For this review, use the dimensioned drawing (mm, ordinates from the lowest corner) and the shaded views. Round coordinates to 2 decimals unless told otherwise and drop trailing zeros. Loops run counter-clockwise (first coordinate to the right, second up) from the corner with the lowest first, then second, coordinate; pieces in that order, holes last. Notation, with made-up numbers: (72, -27.75) -> (112, -27.75) arc R19 ccw to (112, -5.75) -> close; hole circle Ø7 at (37, 70.5). An arc over 180 degrees is marked (long way). Use one line per item in the form item = value. Start each with the question number.
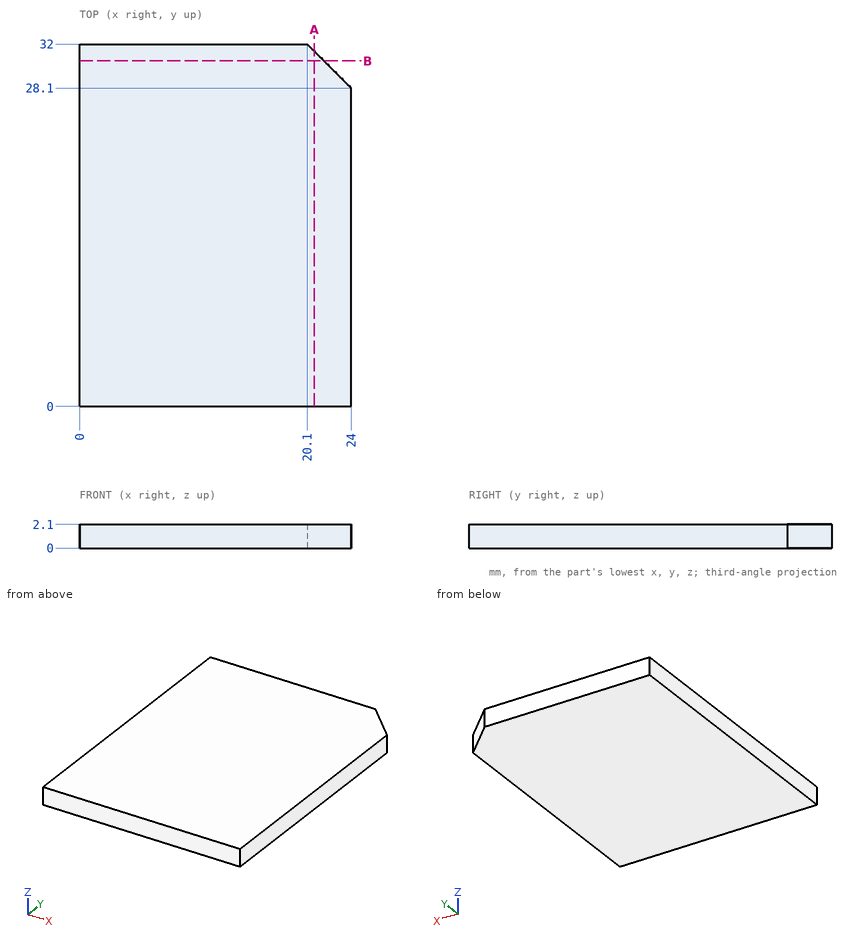
Item 1: Take a section at A-A on x = 20.75. Give the boundary of the cut face in (y, z), plus the area to 3 significant figures.
Item 2: Take a section at B-B on y = 30.5. Give the boundary of the cut face in (x, z).
Item 3: Wall thickness on line 1 (Y direction, x = 22.75, z = 2.05); line 2 (Y direction, x = 22.5, z = 0.3); line 3 (X direction, y = 30, z = 0.3): over which ranges is each line inside the solid? List them lowest first.
Results:
q1.outline = (0, 0) -> (31.35, 0) -> (31.35, 2.1) -> (0, 2.1) -> close
q1.area = 65.8 mm2
q2.outline = (0, 0) -> (21.6, 0) -> (21.6, 2.1) -> (0, 2.1) -> close
q3.line_1 = 0 to 29.35
q3.line_2 = 0 to 29.6
q3.line_3 = 0 to 22.1
